Can you work these out from the model? Positions are in its coordinate system, mm. Face numbers are marked on the shaded views. A direction names the side the tool comes from. Give positions to 0.01 mm unless a question says otherwise; leave off trailing zeros. Loops run counter-clockwise (first coordinate to the right, second up) from the corner with the lowest first, then second, coordinate; pieces in that order, holes last. Notation, with made-up numbers: (-33, 66.5) - (-3, 66.5) arc R17 ccw to (-3, 85.5) - close; hole circle Ø10 at (50, 48.5). An arc over 180 degrees is marked (long way). Write item = value, one per line.
from build123d import *

# Parameters (mm, degrees)
F0_W      = 152.4
F0_H      = 63.5
F1_DEPTH  = 3.81
F2_R      = 8.128
F3_DEPTH  = 3.811
F5_DEPTH  = 10.16
F6_R      = 3.556
F7_DEPTH  = 10.161
F8_R      = 9.525
F9_DEPTH  = 10.16
F10_R     = 9.525
F10_R_2   = 3.556
F11_DEPTH = 10.16
F12_R     = 3.556
F13_DEPTH = 10.161


with BuildPart() as f1:
    # F0 (on Top) → F1 (new body)
    with BuildSketch(Plane.XY):
        with Locations((76.2, 31.75)):
            Rectangle(F0_W, F0_H)
    extrude(amount=F1_DEPTH)

    # F2 (on Top) → F3 (cut, through all)
    with BuildSketch(Plane.XY):
        with Locations((38.1, 12.7)):
            Circle(F2_R)
        with Locations((38.1, 50.8)):
            Circle(F2_R)
        with Locations((76.2, 50.8)):
            Circle(F2_R)
        with Locations((76.2, 12.7)):
            Circle(F2_R)
        with Locations((114.3, 50.8)):
            Circle(F2_R)
        with Locations((114.3, 12.7)):
            Circle(F2_R)
    extrude(amount=F3_DEPTH, mode=Mode.SUBTRACT)

    # F4 (on Top) → F5 (join)
    with BuildSketch(Plane.XY):
        Polygon((59.055, 63.5), (55.245, 63.5), (55.245, 33.655), (20.955, 33.655), (20.955, 63.5), (17.145, 63.5), (17.145, 33.655), (0, 33.655), (0, 29.845), (17.145, 29.845), (17.145, 0), (20.955, 0), (20.955, 29.845), (55.245, 29.845), (55.245, 0), (59.055, 0), (59.055, 29.845), (93.345, 29.845), (93.345, 0), (97.155, 0), (97.155, 29.845), (131.445, 29.845), (131.445, 0), (135.255, 0), (135.255, 29.845), (152.4, 29.845), (152.4, 33.655), (135.255, 33.655), (135.255, 63.5), (131.445, 63.5), (131.445, 33.655), (97.155, 33.655), (97.155, 63.5), (93.345, 63.5), (93.345, 33.655), (59.055, 33.655), align=None)
    extrude(amount=F5_DEPTH)

    # F6 (on Top) → F7 (cut, through all)
    with BuildSketch(Plane.XY):
        with Locations((9.525, 50.8)):
            Circle(F6_R)
        with Locations((9.525, 12.7)):
            Circle(F6_R)
        with Locations((142.875, 12.7)):
            Circle(F6_R)
        with Locations((142.875, 50.8)):
            Circle(F6_R)
    extrude(amount=F7_DEPTH, mode=Mode.SUBTRACT)

    # F8 (on Top) → F9 (join)
    with BuildSketch(Plane.XY):
        with Locations((57.069456, 31.75)):
            Circle(F8_R)
        with Locations((95.169456, 31.75)):
            Circle(F8_R)
        with Locations((19.05, 31.75)):
            Circle(F8_R)
        with Locations((133.269456, 31.75)):
            Circle(F8_R)
    extrude(amount=F9_DEPTH)

    # F10 (on Top) → F11 (join)
    with BuildSketch(Plane.XY):
        with Locations((9.525, 50.8)):
            Circle(F10_R)
        with Locations((9.525, 50.8)):
            Circle(F10_R_2, mode=Mode.SUBTRACT)
        with Locations((9.525, 12.7)):
            Circle(F10_R)
        with Locations((9.525, 12.7)):
            Circle(F10_R_2, mode=Mode.SUBTRACT)
        with Locations((142.875, 50.8)):
            Circle(F10_R)
        with Locations((142.875, 50.8)):
            Circle(F10_R_2, mode=Mode.SUBTRACT)
        with Locations((142.875, 12.7)):
            Circle(F10_R)
        with Locations((142.875, 12.7)):
            Circle(F10_R_2, mode=Mode.SUBTRACT)
    extrude(amount=F11_DEPTH)

    # F12 (on Top) → F13 (cut, through all)
    with BuildSketch(Plane.XY):
        with Locations((19.05, 31.75)):
            Circle(F12_R)
        with Locations((57.15, 31.75)):
            Circle(F12_R)
        with Locations((95.25, 31.75)):
            Circle(F12_R)
        with Locations((133.35, 31.75)):
            Circle(F12_R)
    extrude(amount=F13_DEPTH, mode=Mode.SUBTRACT)


solid = f1.part
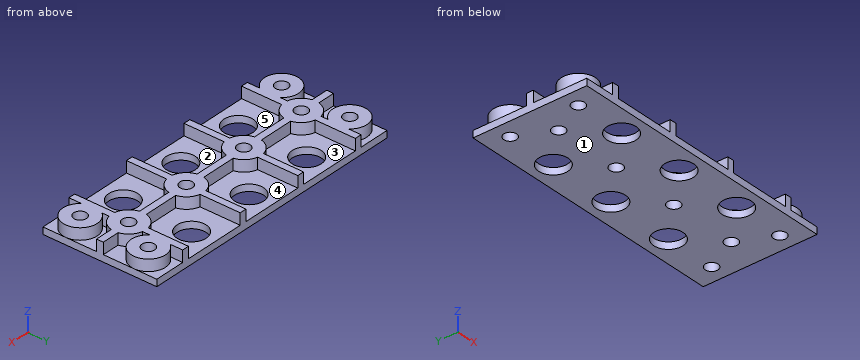
Q1. Imagine slicing it at A-A, the plane x = 95.25. Write out the boundary of the cut face in (y, z).
Output:
outline = (0, 0) - (28.19, 0) - (28.19, 10.16) - (0, 10.16) - close; (35.31, 0) - (63.5, 0) - (63.5, 10.16) - (35.31, 10.16) - close
Q2. For pin 1 (5 mm diameter, centred on y = 18.5, z = 6.5, fed in from -X); pin 2 (5 mm diameter, centred on y = 4, z = 8.5, fed in from +X); pin 3 (4 mm diameter, centred on x = 42.5, z = 3.5, fed in from -Y); pin 4 (1.9 mm diameter, centred on y = 61.5, z = 6, fed in from +X) (3 decimals), each with a flat end and sliding along its axis, tell me the tip position at first contact or that it passes through.
Output:
pin_1 = 0.59
pin_2 = 150.11
pin_3 = 0
pin_4 = 135.255
Q3. Which directions (+Z, -Z, +X, -X, +Y, -Y) give clear straight access to the entire face, cutting with the end or side of a thin tool? Please do the marked faces 4 and 5.
Output:
face_4 = +Z, +Y
face_5 = +Z, -Y
Q4. Imagine slicing it at C-C, the plane x = 38.1. Write out the boundary of the cut face in (y, z) (3 decimals), then the cut area to 3 significant figures.
Output:
outline = (0, 0) - (4.572, 0) - (4.572, 3.81) - (0, 3.81) - close; (20.828, 0) - (42.672, 0) - (42.672, 3.81) - (33.655, 3.81) - (33.655, 10.16) - (29.845, 10.16) - (29.845, 3.81) - (20.828, 3.81) - close; (58.928, 0) - (63.5, 0) - (63.5, 3.81) - (58.928, 3.81) - close
area = 142 mm2
Q5. I need wall thicknesses on L1, parallel to Y at x = 114.3, z = 1.45; L2, parallel to Y at x = 113, z = 1.5; L3, parallel to Y at x = 135.5, z = 6.75. Which ranges of each line are inside material? Lowest first, please.
Output:
L1 = 0 to 4.57, 20.83 to 42.67, 58.93 to 63.5
L2 = 0 to 4.68, 20.72 to 42.78, 58.82 to 63.5
L3 = 6.67 to 18.73, 22.49 to 28.92, 34.58 to 41.01, 44.77 to 56.83
Q6. Imagine slicing it at B-B, the plane y = 31.75. Write out the boundary of the cut face in (x, z).
Output:
outline = (0, 0) - (15.49, 0) - (15.49, 10.16) - (0, 10.16) - close; (22.61, 0) - (53.59, 0) - (53.59, 10.16) - (22.61, 10.16) - close; (60.71, 0) - (91.69, 0) - (91.69, 10.16) - (60.71, 10.16) - close; (98.81, 0) - (129.79, 0) - (129.79, 10.16) - (98.81, 10.16) - close; (136.91, 0) - (152.4, 0) - (152.4, 10.16) - (136.91, 10.16) - close
Q7. Imagine slicing it at D-D, the plane z = 7. Give the number of separate pieces and of enclosed holes in the cut face, then the cut area to 3 significant figures.
Output:
separate_pieces = 1
enclosed_holes = 8
area = 2,870 mm2
Q8. We'd pull the mould along X, two halves only. Please class the marked faces 1, 2 and 3: released by +X, released by -X, zero draft, split by the parting line, or undercut.
Output:
face_1 = zero draft
face_2 = undercut
face_3 = undercut
